Autodesk Inventor part; units mm, degrees
ref_plane "РабПлоскость1" through (89.2173, 100.7825, 86.5043) normal (0, 0, -1) x (-1, 0, 0)
ref_plane "YZ Plane" through (0, 0, 0) normal (1, 0, 0) x (0, 1, 0)
ref_plane "XZ Plane" through (0, 0, 0) normal (0, 1, 0) x (-1, 0, 0)
ref_plane "РабПлоскость1" through (89.2173, 100.7825, 86.5043) normal (0, 0, -1) x (-1, 0, 0)
sketch "Эскиз1" plane through (89.2173, 100.7825, 86.5043) normal (0, 0, -1) x (-1, 0, 0)
  line L0 (0, 7.6342) -> (-13.2857, 7.6342) construction
  line L1 (0, 7.6342) -> (0, 13.6342)
  line L2 (-13.2857, 13.6342) -> (0, 13.6342)
  line L3 (-13.2857, 7.6342) -> (-13.2857, 13.6342)
  line L4 (-26.5714, 7.6342) -> (-39.8571, 7.6342) construction
  line L5 (-26.5714, 7.6342) -> (-26.5714, 13.6342)
  line L6 (-39.8571, 13.6342) -> (-26.5714, 13.6342)
  line L7 (-39.8571, 7.6342) -> (-39.8571, 13.6342)
  line L8 (-53.1429, 7.6342) -> (-66.4286, 7.6342) construction
  line L9 (-53.1429, 7.6342) -> (-53.1429, 13.6342)
  line L10 (-66.4286, 13.6342) -> (-53.1429, 13.6342)
  line L11 (-66.4286, 7.6342) -> (-66.4286, 13.6342)
  line L12 (-79.7143, 7.6342) -> (-93, 7.6342) construction
  line L13 (-79.7143, 7.6342) -> (-79.7143, 13.6342)
  line L14 (-93, 13.6342) -> (-79.7143, 13.6342)
  line L15 (-93, 7.6342) -> (-93, 13.6342)
  line L16 (-13.2857, 7.6342) -> (-26.5714, 7.6342)
  line L17 (-39.8571, 7.6342) -> (-53.1429, 7.6342)
  line L18 (-66.4286, 7.6342) -> (-79.7143, 7.6342)
  line L19 (0, 7.6342) -> (0, -46.3658)
  line L20 (-3, -49.3658) -> (-9.6218, -49.3658)
  line L21 (-93, 7.6342) -> (-93, -46.3658)
  line L22 (-90, -49.3658) -> (-83.3782, -49.3658)
  line L23 (-12.5, -49.3658) -> (-80.5, -49.3658) construction
  arc A0 (-80.3881, -52.1226) -> (-12.6119, -52.1226) centre (-46.5, -49.3658) ccw
  arc A1 (-9.6218, -49.3658) -> (-12.6119, -52.1226) centre (-9.6218, -52.3658) ccw
  arc A2 (-80.3881, -52.1226) -> (-83.3782, -49.3658) centre (-83.3782, -52.3658) ccw
  arc A3 (-93, -46.3658) -> (-90, -49.3658) centre (-90, -46.3658) ccw
  arc A4 (-3, -49.3658) -> (0, -46.3658) centre (-3, -46.3658) ccw
  circle A5 centre (-46.5, -49.2217) radius 6
  circle A6 centre (-62, -42.2217) radius 1.25
  circle A7 centre (-54.25, -55.6451) radius 1.25
  circle A8 centre (-38.75, -55.6451) radius 1.25
  circle A9 centre (-31, -42.2217) radius 1.25
  circle A10 centre (-38.75, -28.7983) radius 1.25
  circle A11 centre (-54.25, -28.7983) radius 1.25
  point P0 (89.2173, -100.7825)
  point P1 (-93, -49.3658)
  dimension "d0" = 57
  dimension "d1" = 34
  dimension "d2" = 3
  dimension "d3" = 6
ref_plane "РабПлоскость2" through (219.2173, 403.7825, -131.4957) normal (0, 0, -1) x (-1, 0, 0)
extrude "Выдавливание1" add sketch "Эскиз1" along normal blind 6
sketch "Эскиз2" plane through (89.2173, 100.7825, 86.5043) normal (0, 0, 1) x (1, 0, 0)
  circle A0 centre (46.5, -42.2217) radius 19
  line L0 (49.5, -2.555) -> (43.5, -2.555)
  line L1 (43.5, -2.555) -> (43.5, -12.8884) construction
  line L2 (43.5, -12.8884) -> (49.5, -12.8884)
  line L3 (49.5, -12.8884) -> (49.5, -2.555) construction
  line L4 (49.5, -12.8884) -> (46.5, -42.2217) construction
  line L5 (46.5, -42.2217) -> (43.5, -12.8884) construction
  line L6 (49.5, -12.8884) -> (43.5, -2.555) construction
  line L7 (43.5, -12.8884) -> (43.5, -23.2217)
  line L8 (43.5, -23.2217) -> (49.5, -23.2217)
  line L9 (49.5, -23.2217) -> (49.5, -12.8884)
  line L10 (43.5, -2.555) -> (43.5, 7.7783)
  line L11 (49.5, -2.555) -> (49.5, 7.7783)
  circle A1 centre (46.5, -7.7217) radius 1.5
  line L12 (18.4286, 7.7783) -> (18.4286, 13.7783) construction
  line L13 (21.4286, 7.7783) -> (21.4286, 13.7783) construction
  line L14 (71.5714, 7.7783) -> (71.5714, 13.7783) construction
  line L15 (74.5714, 7.7783) -> (74.5714, 13.7783) construction
  line L16 (43.5, 7.7783) -> (49.5, 7.7783)
  line L17 (18.4286, 7.7783) -> (18.4286, 1.4283)
  line L18 (18.4286, 1.4283) -> (17.1786, 1.4283)
  line L19 (17.1786, 1.4283) -> (17.1786, -0.8717)
  line L20 (17.1786, -0.8717) -> (18.4286, -0.8717)
  line L21 (18.4286, -0.8717) -> (18.4286, -7.2217)
  line L22 (18.4286, -7.2217) -> (21.4286, -7.2217)
  line L23 (21.4286, -7.2217) -> (21.4286, -0.8717)
  line L24 (21.4286, -0.8717) -> (22.6786, -0.8717)
  line L25 (22.6786, -0.8717) -> (22.6786, 1.4283)
  line L26 (22.6786, 1.4283) -> (21.4286, 1.4283)
  line L27 (21.4286, 1.4283) -> (21.4286, 7.7783)
  line L28 (18.4286, 7.7783) -> (21.4286, 7.7783)
  line L29 (46.5, 7.7783) -> (46.5, -2.555) construction
  line L30 (74.5714, 7.7783) -> (74.5714, 1.4283)
  line L31 (74.5714, 1.4283) -> (75.8214, 1.4283)
  line L32 (75.8214, 1.4283) -> (75.8214, -0.8717)
  line L33 (75.8214, -0.8717) -> (74.5714, -0.8717)
  line L34 (74.5714, -0.8717) -> (74.5714, -7.2217)
  line L35 (74.5714, -7.2217) -> (71.5714, -7.2217)
  line L36 (71.5714, -7.2217) -> (71.5714, -0.8717)
  line L37 (71.5714, -0.8717) -> (70.3214, -0.8717)
  line L38 (70.3214, -0.8717) -> (70.3214, 1.4283)
  line L39 (70.3214, 1.4283) -> (71.5714, 1.4283)
  line L40 (71.5714, 1.4283) -> (71.5714, 7.7783)
  line L41 (71.5714, 7.7783) -> (74.5714, 7.7783)
  line L42 (335, 7.7783) -> (-15, 7.7783) construction
  point P0 (-89.2173, -100.7825)
  dimension "d19" = 6
  dimension "d21" = 3
  dimension "d22" = 5.5
  dimension "d23" = 2.3
  dimension "d26" = 15
extrude "Выдавливание2" cut sketch "Эскиз2" against normal blind 6 contours L8 L7 L2 L9 | L0 L10 L16 L11 | A1 | L28 L27 L26 L25 L24 L23 L22 L21 L20 L19 L18 L17 | L30 L31 L32 L33 L34 L35 L36 L37 L38 L39 L40 L41
sketch "Эскиз4" plane through (168.9316, 114.4167, 86.5043) normal (0, 1, 0) x (1, 0, 0)
  line L0 (13.2857, 6) -> (10.2857, 6)
  line L1 (-79.7143, 0) -> (-79.7143, 6)
  line L2 (13.2857, 6) -> (-79.7143, 6)
  line L3 (-79.7143, 6) -> (-79.7143, 0)
  line L4 (-79.7143, 0) -> (13.2857, 0)
  line L5 (13.2857, 0) -> (13.2857, 6)
  point P0 (-168.9316, 86.5043)
  point P1 (10.2857, 6)
  point P2 (-79.7143, 6)
extrude "Выдавливание3" cut sketch "Эскиз4" against normal blind 1
equation "\"d5\" = d3"
equation "\"d19\" = d3"
equation "\"d14\" = d3"
properties part number "motor3"
Work out the finished part from the listing and answer in its coordinate system (mm). A direction names the side the tool comes from. Round coordinates to 2 decimals unless told otherwise and drop trailing zeros. Write each loop counter-clockwise with the first axis right and the second up, starting at its lowest first coordinate (ties: lowest second). Pieces come first, ordered by that corner, then holes. Notation, with made-up numbers: (-37.75, 44) - (11.25, 44) arc R31 cw to (11.25, 79) - close; hole circle Ø7 at (29.5, 30.5). An arc over 180 degrees is marked (long way). Answer in a Markdown table with one row per item. Add a question column.
1. Given pin 1 (3 mm diameter, centred on x = 96.5, z = 85, fed in from -Y); pin 2 (2 mm diameter, centred on x = 158, z = 85, fed in from +Y); pin 3 (3 mm diameter, centred on x = 127, z = 82, fed in from -Y); pin 4 (3 mm diameter, centred on x = 120.22, y = 58.56, fed in from +Z), each flat-ended and moving along its own axis, determine where each tip first touches the part or whether it passes through.
2. The mould has two halves that part along Y. Classify faces 3 (the flat face through (122, 113.417, 83)), 4 (the flat face through (142.36, 111, 84)), 5 (the cylindrical face through (143.738, 46.358, 83.546)): +Y half, -Y half, draft (parallel to the pull), parting line (faces both ways), or undercut.
3. Find the intervals of material crossed by line 1 along X through (y, z) = (103.5, 83.7); line 2 along X through (y, z) = (100, 81.35); line 3 along X through (y, z) = (95.5, 82.9), in increasing order. Write a range as from..to.
4. For faces 1 (the cylindrical face through (170.585, 50.643, 83.546)), 2 (the flat face through (107.646, 97, 84)), determine the directions among +Z, -Z, +X, -X, +Y, -Y from which every point of the face is accessible in a straight line to the end or side of a thin tool.
5. A cutting plane is placed at A-A, the plane y = 79.5. Determine the outline of the cut face in (x, z).
6. A cutting plane is placed at C-C, the plane x = 143.5. Determine the outline of the cut face in (y, z).
7. A cutting plane is placed at B-B, the plane x = 131. Determine the outline of the cut face in (y, z).
8. A cutting plane is placed at D-D, the plane z = 84.3. Count the separate pieces of the cut face and the enclosed holes in it, and give its area (3 significant figures).
Worked out:
| question | item | result |
|---|---|---|
| 1 | pin 1 | y = 51.42 |
| 1 | pin 2 | y = 108.42 |
| 1 | pin 3 | y = 18.19 |
| 1 | pin 4 | z = 86.5 |
| 2 | face 3 | +Y half |
| 2 | face 4 | draft |
| 2 | face 5 | undercut |
| 3 | line 1 | 89.22..107.65, 110.65..132.72, 138.72..160.79, 163.79..182.22 |
| 3 | line 2 | 89.22..106.4, 111.9..132.72, 138.72..159.54, 165.04..182.22 |
| 3 | line 3 | 89.22..107.65, 110.65..160.79, 163.79..182.22 |
| 4 | face 1 | +Z, -Z, +X, -Y |
| 4 | face 2 | +Z, -Z, +Y |
| 5 | outline | (89.22, 80.5) - (132.72, 80.5) - (132.72, 86.5) - (89.22, 86.5) - close; (138.72, 80.5) - (182.22, 80.5) - (182.22, 86.5) - (138.72, 86.5) - close |
| 6 | outline | (18.32, 80.5) - (43.89, 80.5) - (43.89, 86.5) - (18.32, 86.5) - close; (46.39, 80.5) - (70.73, 80.5) - (70.73, 86.5) - (46.39, 86.5) - close; (73.23, 80.5) - (113.42, 80.5) - (113.42, 86.5) - (73.23, 86.5) - close |
| 7 | outline | (17.75, 80.5) - (47.85, 80.5) - (47.85, 86.5) - (17.75, 86.5) - close; (55.27, 80.5) - (108.42, 80.5) - (108.42, 86.5) - (55.27, 86.5) - close |
| 8 | separate pieces | 1 |
| 8 | enclosed holes | 9 |
| 8 | area | 7,010 mm^2 |
